Work out the finished part from the listing and answer in its coordinate system (mm). A direction names the side the tool comes from. Round coordinates to 2 decimals unless told otherwise and drop trailing zeros. Loops run counter-clockwise (first coordinate to the right, second up) from the corner with the lowest first, then second, coordinate; pieces in that order, holes last. Notation, with made-up numbers: (53, 87) - (64, 87) arc R6 cw to (64, 91) - close; hole circle Ø3 at (59, 81.25). An arc over 180 degrees is marked (long way). Answer as CSV lines item,"result". Start each with the question number.
Q1. Section A-A on z = -22.5 is taken. Write down the section's boundary in (x, y).
Q2. Each of these flat-tipped pins is pushed along its axis until it touches: pin 1 Ø3 at (x, z) = (-1.5, -19) entering from -Y; pin 2 Ø1 at (y, z) = (-1, -17.5) entering from +X; pin 3 Ø0.7 at (y, z) = (0, -1) entering from -X. Where does it stop, or does it pass through?
Q3. The mould has two halves that part along X. Classify faces 3 (the face through (0, 2, -15)), 4 (the face through (2, 2, -2.2)), 5 (the face through (0.63, 1.08, -0.64)): +X half, -X half, draft (parallel to the pull), parting line (faces both ways), or undercut.
Q4. For faces 1 (the face through (0, 0, -27.2)), 2 (the face through (0.616, -1.088, -0.641)), determine the directions among +Z, -Z, +X, -X, +Y, -Y from which every point of the face is accessible in a straight line to the end or side of a thin tool.
Q5. Straight lines are drawn through the part: L1, parallel to Z at x = -1, y = -2.5; L2, parallel to Y at x = 0, z = -10.5; L3, parallel to Y at x = 3, z = -1.25. For each, find the intervals that lie inside material, in ascending order. Write a range as [from, to].
```python
from build123d import *

# Parameters (mm, degrees)
CUT_EXTRUDE2_DEPTH = 1.3


with BuildPart() as part:
    # Sketch1 → Revolve1 (revolve)
    with BuildSketch(Plane(origin=(0, 0, 0), x_dir=(0, 0, -1), z_dir=(1, 0, 0)), mode=Mode.PRIVATE) as revolve1_sk:
        with BuildLine():
            Line((0, 0), (0, 1.435))
            ThreePointArc((0, 1.435), (0.794963972, 2.79089199), (2, 3.8))
            Line((2, 3.8), (2.2, 3.8))
            Line((2.2, 3.8), (2.2, 2.2))
            ThreePointArc((2.2, 2.2), (2.258578644, 2.058578644), (2.4, 2))
            Line((2.4, 2), (26.85, 2))
            Line((26.85, 2), (27.2, 1.65))
            Line((27.2, 1.65), (27.2, 0))
            Line((27.2, 0), (0, 0))
        make_face()
    revolve(revolve1_sk.sketch.rotate(Axis((0, 0, 0), (0, 0, -1)), 90), axis=Axis((0, 0, 0), (0, 0, -1)))

    # Sketch2 → Cut-Extrude2 (cut)
    with BuildSketch(Plane.XY):
        Polygon((0, -1.443375673), (1.25, -0.721687836), (1.25, 0.721687836), (0, 1.443375673), (-1.25, 0.721687836), (-1.25, -0.721687836), align=None)
    extrude(amount=-CUT_EXTRUDE2_DEPTH, mode=Mode.SUBTRACT)

    # Sketch5 → Cut-Revolve3 (revolve, cut)
    with BuildSketch(Plane(origin=(0, 0, 0), x_dir=(0, 0, -1), z_dir=(1, 0, 0)), mode=Mode.PRIVATE) as cut_revolve3_sk:
        Polygon((0.049570601, -1.25), (0, -1.435), (0, -1.25), align=None)
    revolve(cut_revolve3_sk.sketch.rotate(Axis((0, 0, 0), (0, 0, -1)), 119.415596887), axis=Axis((0, 0, 0), (0, 0, -1)), mode=Mode.SUBTRACT)

    # Sketch4 → Cut-Revolve2 (revolve, cut)
    with BuildSketch(Plane(origin=(0, 0, 0), x_dir=(0, 0, -1), z_dir=(1, 0, 0)), mode=Mode.PRIVATE) as cut_revolve2_sk:
        Polygon((1.3, 0), (1.3, -1.443375673), (2.133333333, 0), align=None)
    revolve(cut_revolve2_sk.sketch.rotate(Axis((0, 0, -1.3), (0, 0, -1)), 119.415596887), axis=Axis((0, 0, -1.3), (0, 0, -1)), mode=Mode.SUBTRACT)


solid = part.part
```
Findings:
1,outline,"circle Ø4 at (0, 0)"
2,pin 1,"stops at y = -2"
2,pin 2,"stops at x = 1.94"
2,pin 3,"stops at x = -3.34"
3,face 3,"parting line"
3,face 4,"draft"
3,face 5,"undercut"
4,face 1,"-Z, +X, -X, +Y, -Y"
4,face 2,"+Z"
5,L1,"z = [-2.2, -0.71]"
5,L2,"y = [-2, 2]"
5,L3,"y = [-1.27, 1.27]"
